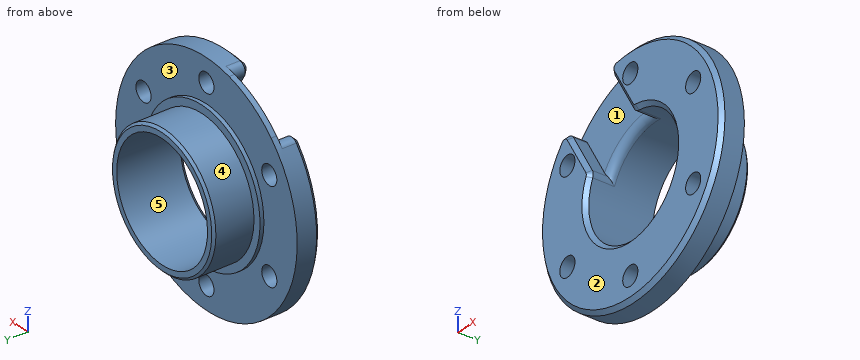
from build123d import *

# Parameters (mm, degrees)
SKETCH_1_R          = 15
SKETCH_1_R_2        = 7.5
SKETCH_1_R_3        = 1
EXTRUDE_1_DEPTH     = 3
SKETCH_2_R          = 8.5
SKETCH_2_R_2        = 7.5
EXTRUDE_2_DEPTH     = 5.7
SKETCH_3_R          = 9.5
SKETCH_3_R_2        = 8.5
EXTRUDE_3_DEPTH     = 0.5
HOLE_WIZARD_M3_1_D  = 2.5
CHAMFER_2_SIZE      = 0.3
CUT_EXTRUDE_2_DEPTH = 2.3
FILLET_START        = -1
FILLET_2_DEPTH      = 4.3000001
FILLET_2_2_DEPTH    = 3.3
FILLET_START_2      = 2.3
FILLET_2_3_DEPTH    = 0.7
CHAMFER_3_SIZE      = 0.5


with BuildPart() as part:
    # Sketch 1 → Extrude 1 (new body)
    with BuildSketch(Plane(origin=(0, 0, 0), x_dir=(1, 0, 0), z_dir=(0, 1, 0))):
        with Locations(Location((0, 0, 0), (0, 0, 270))):
            Circle(SKETCH_1_R)
        with Locations(Location((0, 0, 0), (0, 0, 270))):
            Circle(SKETCH_1_R_2, mode=Mode.SUBTRACT)
        with Locations(Location((0, 12, 0), (0, 0, 270))):
            Circle(SKETCH_1_R_3, mode=Mode.SUBTRACT)
        with Locations(Location((10.392304845, 6, 0), (0, 0, 270))):
            Circle(SKETCH_1_R_3, mode=Mode.SUBTRACT)
        with Locations(Location((10.392304845, -6, 0), (0, 0, 270))):
            Circle(SKETCH_1_R_3, mode=Mode.SUBTRACT)
        with Locations(Location((0, -12, 0), (0, 0, 270))):
            Circle(SKETCH_1_R_3, mode=Mode.SUBTRACT)
        with Locations(Location((-10.392304845, -6, 0), (0, 0, 270))):
            Circle(SKETCH_1_R_3, mode=Mode.SUBTRACT)
        with Locations(Location((-10.392304845, 6, 0), (0, 0, 270))):
            Circle(SKETCH_1_R_3, mode=Mode.SUBTRACT)
    extrude(amount=EXTRUDE_1_DEPTH)

    # Sketch 2 → Extrude 2 (add)
    with BuildSketch(Plane(origin=(0, 3, 0), x_dir=(1, 0, 0), z_dir=(0, 1, 0))):
        with Locations(Location((0, 0, 0), (0, 0, 270))):
            Circle(SKETCH_2_R)
        with Locations(Location((0, 0, 0), (0, 0, 270))):
            Circle(SKETCH_2_R_2, mode=Mode.SUBTRACT)
    extrude(amount=EXTRUDE_2_DEPTH)

    # Sketch 3 → Extrude 3 (add)
    with BuildSketch(Plane(origin=(0, 3, 0), x_dir=(1, 0, 0), z_dir=(0, 1, 0))):
        with Locations(Location((0, 0, 0), (0, 0, 270))):
            Circle(SKETCH_3_R)
        with Locations(Location((0, 0, 0), (0, 0, 270))):
            Circle(SKETCH_3_R_2, mode=Mode.SUBTRACT)
    extrude(amount=EXTRUDE_3_DEPTH)

    # Hole Wizard M3 _1 (through all)
    with Locations(Plane(origin=(0, 0, 0), x_dir=(-1, 0, 0), z_dir=(0, -1, 0))):
        with Locations((0, 12), (10.392304845, 6), (10.392304845, -6), (0, -12), (-10.392304845, -6), (-10.392304845, 6)):
            Hole(HOLE_WIZARD_M3_1_D / 2)

    # Chamfer 2
    chamfer_2_edges = [part.edges().sort_by_distance(p)[0] for p in [
        (0, 8.7, -8.5),
    ]]
    chamfer(chamfer_2_edges, length=CHAMFER_2_SIZE)

    # Sketch 7 → Cut-Extrude 2 (cut)
    with BuildSketch(Plane.XZ):
        with BuildLine():
            Line((-3.464101615, -2), (-12.464101615, 13.588457268))
            ThreePointArc((-12.464101615, 13.588457268), (-11, 19.052558883), (-5.535898385, 17.588457268))
            Line((-5.535898385, 17.588457268), (3.464101615, 2))
            ThreePointArc((3.464101615, 2), (2, -3.464101615), (-3.464101615, -2))
        make_face()
    extrude(amount=-CUT_EXTRUDE_2_DEPTH, mode=Mode.SUBTRACT)

    # Fillet 2: read off the stored shape, not the designer's step
    # Fillet 2 outline → Fillet 2 (cut)
    with BuildSketch(Plane(origin=(0, 0, 0), x_dir=(1, 0, 0), z_dir=(0, 1, 0)).offset(FILLET_START)):
        with BuildLine():
            ThreePointArc((0.788113454, -7.458476868), (-3.75, -6.495190528), (-6.853287168, -3.046712162))
            ThreePointArc((-6.853287168, -3.046712162), (-6.768443854, -3.50555422), (-6.901033386, -3.95294045))
            Line((-6.901033386, -3.95294045), (-10.692517763, -10.519984026))
            ThreePointArc((-10.692517763, -10.519984026), (-7.5, -12.990381057), (-3.764314532, -14.519984026))
            Line((-3.764314532, -14.519984026), (0.027169844, -7.95294045))
            ThreePointArc((0.027169844, -7.95294045), (0.348322918, -7.614421432), (0.788113454, -7.458476868))
        make_face()
    extrude(amount=FILLET_2_DEPTH, mode=Mode.SUBTRACT)

    # Fillet 2 2 outline → Fillet 2 2 (cut)
    with BuildSketch(Plane(origin=(0, 0, 0), x_dir=(1, 0, 0), z_dir=(0, 1, 0)).offset(FILLET_START)):
        with BuildLine():
            ThreePointArc((-2.365951496, -14.812233914), (-3.111088885, -14.254670597), (-3.0742468, -13.324751653))
            Line((-3.0742468, -13.324751653), (-3.764314532, -14.519984026))
            ThreePointArc((-3.764314532, -14.519984026), (-3.068614165, -14.682765649), (-2.365951496, -14.812233914))
        make_face()
        with BuildLine():
            ThreePointArc((-11.644795108, -9.455091057), (-11.181340967, -9.998880646), (-10.692517763, -10.519984026))
            Line((-10.692517763, -10.519984026), (-10.00245003, -9.324751653))
            ThreePointArc((-10.00245003, -9.324751653), (-10.789362416, -9.821617306), (-11.644795108, -9.455091057))
        make_face()
    extrude(amount=FILLET_2_2_DEPTH, mode=Mode.SUBTRACT)

    # Fillet 2 3 outline → Fillet 2 3 (add)
    with BuildSketch(Plane(origin=(0, 0, 0), x_dir=(1, 0, 0), z_dir=(0, 1, 0)).offset(FILLET_START_2)):
        with BuildLine():
            Line((-7.7725236, -5.462405778), (-10.692517763, -10.519984025))
            ThreePointArc((-10.692517763, -10.519984025), (-7.5, -12.990381057), (-3.764314532, -14.519984026))
            Line((-3.764314532, -14.519984026), (-0.84432037, -9.462405778))
            ThreePointArc((-0.84432037, -9.462405778), (-4.75, -8.227241336), (-7.7725236, -5.462405778))
        make_face()
    extrude(amount=FILLET_2_3_DEPTH)

    # Fillet 2 4 outline → Fillet 2 4 (revolve)
    with BuildSketch(Plane.XY):
        with BuildLine():
            Line((9.5, 2.3), (9.5, 3.3000001))
            Line((9.5, 3.3000001), (7.5, 3.3))
            ThreePointArc((7.5, 3.3), (7.792893219, 2.592893219), (8.5, 2.3))
            Line((8.5, 2.3), (9.5, 2.3))
        make_face()
    revolve(axis=Axis((0, 0, 0), (0, 1, 0)))

    # Chamfer 3
    chamfer_3_edges = [part.edges().sort_by_distance(p)[0] for p in [
        (3.75, 0, -6.495190528),
        (-1.523538478, 0, 10.638846051),
        (-8.451741708, 0, 6.638846051),
        (7.5, 0, -12.990381057),
        (-10.789362416, 0, 9.821617306),
        (-3.111088885, 0, 14.254670597),
        (-6.768443854, 0, 3.50555422),
        (0.348322918, 0, 7.614421432),
    ]]
    chamfer(chamfer_3_edges, length=CHAMFER_3_SIZE)


solid = part.part
Verification items for the finished model (mm, model axes). Face numbers are marked on the shaded views. A direction names the side the tool comes from. Round coordinates to 2 decimals unless told otherwise and drop trailing zeros. Loops run counter-clockwise (first coordinate to the right, second up) from the corner with the lowest first, then second, coordinate; pieces in that order, holes last. Notation, with made-up numbers: (69, -36) - (101, -36) arc R16 ccw to (101, -7) - close; hole circle Ø10 at (-1.75, 29). An arc over 180 degrees is marked (long way). Use a Markdown table: item, result. Add a question column.
1. Access from +Z, -Z, +X, -X, +Y, -Y to the whole of each face (thin tool, end or side, straight path). Record for the marked faces 1 and 2.
2. Section check B-B, the plane y = 4.25. Record the boundary of the cut face in (x, z), plus the area to 3 significant figures.
3. Section check C-C, the plane z = 6. Give the number of separate pieces and of enclosed holes in the cut face, plus the area to 3 significant figures.
4. Gauge pin test, flat ends, axial feed: pin 1 (4 mm diameter, centred on x = 11.5, z = -12, fed in from +Y); pin 2 (5.5 mm diameter, centred on x = -3, z = -3, fed in from +Y); pin 3 (2 mm diameter, centred on y = 1.5, z = 10, fed in from +X). Record the tip position at first contact, or that the pin passes through.
5. Release check for a two-part mould opening along X. For the marked faces 3, 4 and 5 record: released by +X, released by -X, zero draft, split by the parting line, or undercut.
6. Thickness scan on probe 1 along X at (y, z) = (1.25, -6); probe 2 along Z at (x, y) = (0, 2.5); probe 3 along X at (y, z) = (1.95, 6). Record the ranges inside material, lowest first. Write a range as [from, to].
7. Section check A-A, the plane z = 0. Record the boundary of the cut face in (x, y), plus the area to 3 significant figures.
Checks:
| question | item | result |
|---|---|---|
| 1 | face 1 | -Y |
| 1 | face 2 | +Z, -Z, +X, -X, -Y |
| 2 | outline | circle Ø17 at (0, 0); hole circle Ø15 at (0, 0) |
| 2 | area | 50.3 mm^2 |
| 3 | separate pieces | 4 |
| 3 | enclosed holes | 0 |
| 3 | area | 49.8 mm^2 |
| 4 | pin 1 | stops at y = 3 |
| 4 | pin 2 | passes through |
| 4 | pin 3 | stops at x = 12 |
| 5 | face 3 | zero draft |
| 5 | face 4 | split by the parting line |
| 5 | face 5 | undercut |
| 6 | probe 1 | x = [-13.75, -11.64], [-9.14, -4.5], [4.5, 9.14], [11.64, 13.75] |
| 6 | probe 2 | z = [-15, -13.25], [-10.75, -7.5], [7.9, 10.75], [13.25, 15] |
| 6 | probe 3 | x = [-13.75, -11.64], [-9.14, -8.08], [4.5, 9.14], [11.64, 13.75] |
| 7 | outline | (-15, 0.5) - (-14.5, 0) - (-8, 0) - (-7.5, 0.5) - (-7.5, 8.7) - (-8.2, 8.7) - (-8.5, 8.4) - (-8.5, 3.5) - (-9.5, 3.5) - (-9.5, 3) - (-15, 3) - close; (7.5, 0.5) - (8, 0) - (14.5, 0) - (15, 0.5) - (15, 3) - (9.5, 3) - (9.5, 3.5) - (8.5, 3.5) - (8.5, 8.4) - (8.2, 8.7) - (7.5, 8.7) - close |
| 7 | area | 56.8 mm^2 |
